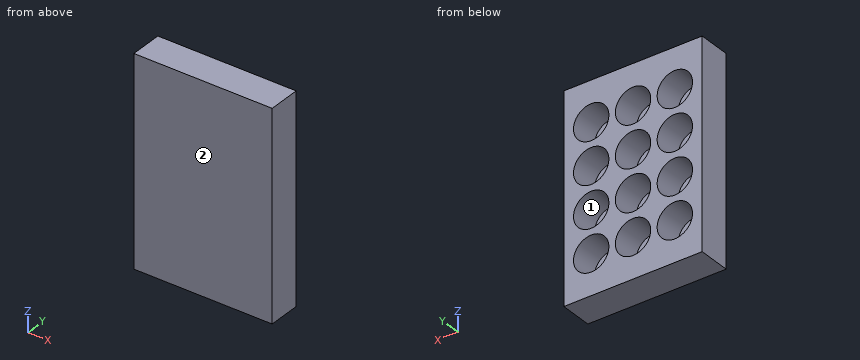
from build123d import *

# Parameters (mm, degrees)
SKETCH1_W            = 86
SKETCH1_H            = 128
BOSS_EXTRUDE1_DEPTH  = 20.2
SKETCH2_R            = 11
CUT_EXTRUDE1_DEPTH   = 17.7
LPATTERN3_COUNT      = 4
LPATTERN3_PITCH      = 26
LPATTERN3_COUNT_DIR2 = 3
LPATTERN3_PITCH_DIR2 = 26


with BuildPart() as part:
    # Sketch1 → Boss-Extrude1 (new body)
    with BuildSketch(Plane(origin=(0, 0, 0), x_dir=(1, 0, 0), z_dir=(0, 1, 0))):
        with Locations((43, 64)):
            Rectangle(SKETCH1_W, SKETCH1_H)
    extrude(amount=BOSS_EXTRUDE1_DEPTH)

    # Sketch2 → Cut-Extrude1 (cut)
    with BuildSketch(Plane(origin=(0, 20.2, 0), x_dir=(1, 0, 0), z_dir=(0, 1, 0))):
        with Locations((17, 25)):
            Circle(SKETCH2_R)
    cut_extrude1 = extrude(amount=-CUT_EXTRUDE1_DEPTH, mode=Mode.SUBTRACT)

    # LPattern3: Cut-Extrude1 4 × 3
    with Locations(*[(j * LPATTERN3_PITCH_DIR2, 0, -i * LPATTERN3_PITCH) for i in range(LPATTERN3_COUNT) for j in range(LPATTERN3_COUNT_DIR2) if (i, j) != (0, 0)]):
        add(cut_extrude1, mode=Mode.SUBTRACT)


solid = part.part
Can you work these out from the model? Positions are in its coordinate system, mm. Face numbers are marked on the shaded views. A direction names the side the tool comes from. Give positions to 0.01 mm unless a question says otherwise; leave off trailing zeros. Order: outer loops, then holes, each group sorted by start corner. A loop starts at its lowest first (then second) coordinate and runs counter-clockwise, first axis right, second up. Notation, with made-up numbers: M 67.5,54 L 79.5,54 A22 ccw 79.5,78 Z; hole C 15,40 d7. An arc over 180 degrees is marked long. Use one line per item in the form item = value. Start each with the question number.
Item 1: If we section it at C-C (z = -51): Write out the boundary of the cut face in (x, y).
Item 2: For the marked faces 1 and 2, which set-ups out of +Z, -Z, +X, -X, +Y, -Y let a thin tool reach every point of the face, with its end or its side?
Item 3: If I drill on line 1 along Z through (x, y) = (17, 11.25); line 2 along X through (y, z) = (15.5, -103); line 3 along Z through (x, y) = (15, 17.75), over which ranges is the centre line in solid material (lowest first)?
Item 4: If we section it at D-D (x = 11): Write out the boundary of the cut face in (y, z).
Item 5: Will this pin go through, and if not, where does the flat tip stop? pin 1 Ø13 at (x, z) = (69, -51) entering from +Y.
Item 6: If we section it at A-A (y = 17.75): State how many separate pieces and enclosed holes the cut face has, then the cut area to 3 significant figures.
Item 7: If we section it at B-B (x = 43): Write out the boundary of the cut face in (y, z), then the cut area to 3 significant figures.
Outcome:
q1.outline = M 0,0 L 86,0 L 86,20.2 L 80,20.2 L 80,2.5 L 58,2.5 L 58,20.2 L 54,20.2 L 54,2.5 L 32,2.5 L 32,20.2 L 28,20.2 L 28,2.5 L 6,2.5 L 6,20.2 L 0,20.2 Z
q2.face_1 = +Y
q2.face_2 = +Z, -Z, +X, -X, -Y
q3.line_1 = -128 to -114, -92 to -88, -66 to -62, -40 to -36, -14 to 0
q3.line_2 = 0 to 6, 28 to 32, 54 to 58, 80 to 86
q3.line_3 = -128 to -113.82, -92.18 to -87.82, -66.18 to -61.82, -40.18 to -35.82, -14.18 to 0
q4.outline = M 0,-128 L 20.2,-128 L 20.2,-112.22 L 2.5,-112.22 L 2.5,-93.78 L 20.2,-93.78 L 20.2,-86.22 L 2.5,-86.22 L 2.5,-67.78 L 20.2,-67.78 L 20.2,-60.22 L 2.5,-60.22 L 2.5,-41.78 L 20.2,-41.78 L 20.2,-34.22 L 2.5,-34.22 L 2.5,-15.78 L 20.2,-15.78 L 20.2,0 L 0,0 Z
q5.pin_1 = 2.5
q6.separate_pieces = 1
q6.enclosed_holes = 12
q6.area = 6,450 mm2
q7.outline = M 0,-128 L 20.2,-128 L 20.2,-114 L 2.5,-114 L 2.5,-92 L 20.2,-92 L 20.2,-88 L 2.5,-88 L 2.5,-66 L 20.2,-66 L 20.2,-62 L 2.5,-62 L 2.5,-40 L 20.2,-40 L 20.2,-36 L 2.5,-36 L 2.5,-14 L 20.2,-14 L 20.2,0 L 0,0 Z
q7.area = 1,030 mm2
